```python
from build123d import *

# Parameters (mm, degrees)
SKETCH2_R           = 1.6
SKETCH2_R_2         = 1.5
SKETCH2_W           = 25.4
SKETCH2_H           = 46
BOSS_EXTRUDE1_DEPTH = 2
SKETCH5_R           = 1.6
SKETCH5_R_2         = 2.25
SKETCH5_W           = 25.4
SKETCH5_H           = 46
BOSS_EXTRUDE3_DEPTH = 3
SKETCH2_4_W         = 10
SKETCH2_4_H         = 30
SKETCH2_4_H_2       = 70
BOSS_EXTRUDE4_DEPTH = 5
CHAMFER1_SIZE       = 1.75
SKETCH7_R           = 2.05
CUT_EXTRUDE1_DEPTH  = 9


with BuildPart() as part:
    # Sketch2 → Boss-Extrude1 (new body)
    with BuildSketch(Plane(origin=(0, 0, 0), x_dir=(1, 0, 0), z_dir=(0, 1, 0))):
        Polygon((9.15, 64.2), (-37.8, 64.2), (-37.8, -65.8), (9.15, -65.8), (37.8, -65.8), (37.8, 64.2), align=None)
        with Locations((-7.45, -62.2)):
            Circle(SKETCH2_R, mode=Mode.SUBTRACT)
        with Locations((-7.45, -42.2)):
            Circle(SKETCH2_R, mode=Mode.SUBTRACT)
        with Locations((-15, -17)):
            Circle(SKETCH2_R_2, mode=Mode.SUBTRACT)
        with Locations((-8.5, -23.3)):
            Circle(SKETCH2_R_2, mode=Mode.SUBTRACT)
        with BuildLine():
            ThreePointArc((5.95, -62.2), (7.55, -60.6), (9.15, -62.2))
            ThreePointArc((9.15, -62.2), (7.55, -63.8), (5.95, -62.2))
        make_face(mode=Mode.SUBTRACT)
        with BuildLine():
            ThreePointArc((5.95, -42.2), (7.55, -40.6), (9.15, -42.2))
            ThreePointArc((9.15, -42.2), (7.55, -43.8), (5.95, -42.2))
        make_face(mode=Mode.SUBTRACT)
        with Locations((8.5, -23.3)):
            Circle(SKETCH2_R_2, mode=Mode.SUBTRACT)
        with Locations((15, -17)):
            Circle(SKETCH2_R_2, mode=Mode.SUBTRACT)
        with Locations((-15, 0)):
            Circle(SKETCH2_R_2, mode=Mode.SUBTRACT)
        with Locations((-15, 17)):
            Circle(SKETCH2_R_2, mode=Mode.SUBTRACT)
        with Locations((-7.45, 40.6)):
            Circle(SKETCH2_R, mode=Mode.SUBTRACT)
        with Locations((-7.45, 60.6)):
            Circle(SKETCH2_R, mode=Mode.SUBTRACT)
        with Locations((0, 2)):
            Rectangle(SKETCH2_W, SKETCH2_H, mode=Mode.SUBTRACT)
        with Locations((15, 0)):
            Circle(SKETCH2_R_2, mode=Mode.SUBTRACT)
        with Locations((15, 17)):
            Circle(SKETCH2_R_2, mode=Mode.SUBTRACT)
        with BuildLine():
            ThreePointArc((7.55, 39), (6.41862915, 39.46862915), (5.95, 40.6))
            ThreePointArc((5.95, 40.6), (8.68137085, 41.73137085), (7.55, 39))
        make_face(mode=Mode.SUBTRACT)
        with Locations((7.55, 60.6)):
            Circle(SKETCH2_R, mode=Mode.SUBTRACT)
    extrude(amount=BOSS_EXTRUDE1_DEPTH)

    # Sketch5 → Boss-Extrude3 (add)
    with BuildSketch(Plane.XZ):
        Polygon((37.8, 30.8), (37.8, 65.8), (-37.8, 65.8), (-37.8, 30.8), (-37.8, -29.2), (-37.8, -64.2), (37.8, -64.2), (37.8, -29.2), align=None)
        with Locations((-7.45, -60.6)):
            Circle(SKETCH5_R, mode=Mode.SUBTRACT)
        with Locations((-7.45, -40.6)):
            Circle(SKETCH5_R, mode=Mode.SUBTRACT)
        with Locations((-15, -17)):
            Circle(SKETCH5_R_2, mode=Mode.SUBTRACT)
        with Locations((-15, 0)):
            Circle(SKETCH5_R_2, mode=Mode.SUBTRACT)
        with Locations((0, -2)):
            Rectangle(SKETCH5_W, SKETCH5_H, mode=Mode.SUBTRACT)
        with Locations((7.55, -60.6)):
            Circle(SKETCH5_R, mode=Mode.SUBTRACT)
        with Locations((7.55, -40.6)):
            Circle(SKETCH5_R, mode=Mode.SUBTRACT)
        with Locations((15, -17)):
            Circle(SKETCH5_R_2, mode=Mode.SUBTRACT)
        with Locations((15, 0)):
            Circle(SKETCH5_R_2, mode=Mode.SUBTRACT)
        with Locations((-15, 17)):
            Circle(SKETCH5_R_2, mode=Mode.SUBTRACT)
        with Locations((-8.5, 23.3)):
            Circle(SKETCH5_R_2, mode=Mode.SUBTRACT)
        with Locations((-7.45, 42.2)):
            Circle(SKETCH5_R, mode=Mode.SUBTRACT)
        with Locations((-7.45, 62.2)):
            Circle(SKETCH5_R, mode=Mode.SUBTRACT)
        with Locations((15, 17)):
            Circle(SKETCH5_R_2, mode=Mode.SUBTRACT)
        with Locations((8.5, 23.3)):
            Circle(SKETCH5_R_2, mode=Mode.SUBTRACT)
        with Locations((7.55, 42.2)):
            Circle(SKETCH5_R, mode=Mode.SUBTRACT)
        with Locations((7.55, 62.2)):
            Circle(SKETCH5_R, mode=Mode.SUBTRACT)
    extrude(amount=BOSS_EXTRUDE3_DEPTH)

    # Sketch2_4 → Boss-Extrude4 (add)
    with BuildSketch(Plane(origin=(0, 0, 0), x_dir=(1, 0, 0), z_dir=(0, 1, 0))):
        with Locations((27.8, 49.2)):
            Rectangle(SKETCH2_4_W, SKETCH2_4_H)
        with Locations((27.8, -0.8)):
            Rectangle(SKETCH2_4_W, SKETCH2_4_H_2)
        with Locations((27.8, -50.8)):
            Rectangle(SKETCH2_4_W, SKETCH2_4_H)
        with Locations((-27.8, 49.2)):
            Rectangle(SKETCH2_4_W, SKETCH2_4_H)
        with Locations((-27.8, -0.8)):
            Rectangle(SKETCH2_4_W, SKETCH2_4_H_2)
        with Locations((-27.8, -50.8)):
            Rectangle(SKETCH2_4_W, SKETCH2_4_H)
    extrude(amount=BOSS_EXTRUDE4_DEPTH)

    # Chamfer1
    chamfer1_edges = [part.edges().sort_by_distance(p)[0] for p in [
        (-9.05, 2, 42.2),
        (9.15, 2, 42.2),
        (9.15, 2, 62.2),
        (-9.05, 2, 62.2),
        (-9.05, 2, -40.6),
        (-9.05, 2, -60.6),
        (5.95, 2, -60.6),
        (7.55, 2, -42.2),
    ]]
    chamfer(chamfer1_edges, length=CHAMFER1_SIZE)

    # Sketch7 → Cut-Extrude1 (cut, through all)
    with BuildSketch(Plane(origin=(0, 5, 0), x_dir=(1, 0, 0), z_dir=(0, 1, 0))):
        with Locations((-27.8, -0.8)):
            Circle(SKETCH7_R)
    extrude(amount=-CUT_EXTRUDE1_DEPTH, mode=Mode.SUBTRACT)


solid = part.part
```
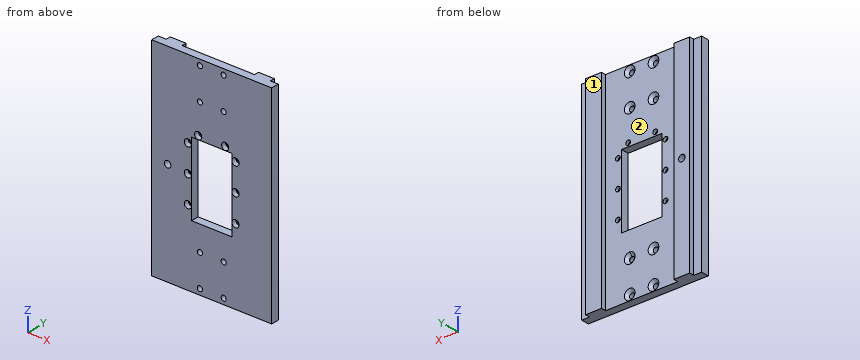
Geometry check sheet. Reference: the model listing, model coordinates, mm. Face numbers are marked on the shaded views. Coordinates: 2 decimals unless noted, no trailing zeros. Write each loop counter-clockwise with the first axis right and the second up, starting at its lowest first coordinate (ties: lowest second). Pieces come first, ordered by that corner, then holes. Notation, with made-up numbers: M 35,1 L 56,1 A21 cw 56,12 Z; hole C 36.25,-18.75 d10. An arc over 180 degrees is marked long. Use one line per item in the form item = value. Start each with the question number.
1) Thickness scan on probe 1 along X at (y, z) = (1.45, 23.3); probe 2 along Z at (x, y) = (15, -2.05); probe 3 along X at (y, z) = (-2, -22). Record the ranges inside material, lowest first. Write a range as from..to.
2) Section check A-A on x = -27.8. Enter the section's corners in (y, z), and give its area (3 significant figures).
3) Section check B-B on z = -60.6. Enter the section's corners in (x, y).
4) Section check C-C on y = -1.5. State how many separate pieces and enclosed holes the cut face has, and give its area (3 significant figures).
5) Release check for a two-part mould opening along X. For the marked faces 1 and 2 record: pulls with the +X half, pulls with the -X half, needs draft (parallel to the pull), parting line crosses it, or undercut.
6) Section check D-D on z = -4.5. Enter the section's corners in (x, y).
7) Go/stop test with flat-tipped pins: pin 1 Ø1.3 at (x, z) = (14.5, -16.5) entering from -Y; pin 2 Ø3.5 at (x, z) = (-15, 0) entering from -Y; pin 3 Ø5 at (x, z) = (-7.45, 42.2) entering from +Y; pin 4 Ø5 at (x, z) = (-15, 17) entering from +Y. Record where each tip stops, or that it passes through.
Responses:
q1.probe_1 = -37.8..-10, -7..7, 10..37.8
q1.probe_2 = -64.2..-19.25, -14.75..-2.25, 2.25..14.75, 19.25..65.8
q1.probe_3 = -37.8..-12.7, 12.7..37.8
q2.outline = M -3,-64.2 L 5,-64.2 L 5,-1.25 L -3,-1.25 Z; M -3,2.85 L 5,2.85 L 5,65.8 L -3,65.8 Z
q2.area = 1,010 mm2
q3.outline = M -37.8,-3 L -9.05,-3 L -9.05,0.25 L -10.8,2 L -22.8,2 L -22.8,5 L -32.8,5 L -32.8,2 L -37.8,2 Z; M -5.85,-3 L 5.95,-3 L 5.95,0.25 L 4.2,2 L -4.1,2 L -5.85,0.25 Z; M 9.15,-3 L 37.8,-3 L 37.8,2 L 32.8,2 L 32.8,5 L 22.8,5 L 22.8,2 L 10.9,2 L 9.15,0.25 Z
q4.separate_pieces = 1
q4.enclosed_holes = 18
q4.area = 8,450 mm2
q5.face_1 = needs draft
q5.face_2 = undercut
q6.outline = M -37.8,-3 L -12.7,-3 L -12.7,2 L -22.8,2 L -22.8,5 L -32.8,5 L -32.8,2 L -37.8,2 Z; M 12.7,-3 L 37.8,-3 L 37.8,2 L 32.8,2 L 32.8,5 L 22.8,5 L 22.8,2 L 12.7,2 Z
q7.pin_1 = through
q7.pin_2 = 0
q7.pin_3 = 1.15
q7.pin_4 = 2
